Check sheet for the modelled part. Datum: model origin and axes. Units: mm. A direction names the side the tool comes from. Give positions to 0.01 mm unless a question says otherwise; leave off trailing zeros. Order: outer loops, then holes, each group sorted by start corner. A loop starts at its lowest first (then second) coordinate and runs counter-clockwise, first axis right, second up. Notation, with made-up numbers: (79.5, -28) -> (89.5, -28) arc R12 ccw to (89.5, -7) -> close; hole circle Ø5 at (13, 16). An arc over 180 degrees is marked (long way). One line per question, with ' | ' between items.
```python
from build123d import *

# Parameters (mm, degrees)
BOSS_EXTRUDE1_DEPTH = 350
BOSS_EXTRUDE2_DEPTH = 250
BOSS_EXTRUDE3_START = 250
BOSS_EXTRUDE3_DEPTH = 250
BOSS_EXTRUDE4_START = 350
SKETCH2_5_W         = 700
SKETCH2_5_H         = 50
BOSS_EXTRUDE4_DEPTH = 350
SKETCH3_R           = 100
CUT_EXTRUDE1_DEPTH  = 25


with BuildPart() as part:
    # Sketch2 → Boss-Extrude1 (new body)
    with BuildSketch(Plane.XY):
        with BuildLine():
            ThreePointArc((-86.602540378, -50), (-96.592582629, -25.88190451), (-100, 0))
            Line((-100, 0), (-720, 0))
            Line((-720, 0), (-720, -50))
            Line((-720, -50), (-86.602540378, -50))
        make_face()
        with BuildLine():
            Line((-20, 0), (-100, 0))
            ThreePointArc((-100, 0), (-96.592582629, -25.88190451), (-86.602540378, -50))
            Line((-86.602540378, -50), (-20, -50))
            Line((-20, -50), (-20, 0))
        make_face()
        with BuildLine():
            Line((0, 1020), (-50, 1020))
            Line((-50, 1020), (-100, 1020))
            ThreePointArc((-100, 1020), (-32.986729188, 522.100663541), (-50, 20))
            Line((-50, 20), (50, 20))
            ThreePointArc((50, 20), (67.013270812, 522.100663541), (0, 1020))
        make_face()
    extrude(amount=-BOSS_EXTRUDE1_DEPTH)

    # Sketch2_3 → Boss-Extrude2 (add)
    with BuildSketch(Plane.XY):
        with BuildLine():
            Line((0, 20), (0, -100))
            ThreePointArc((0, -100), (70.710678119, -70.710678119), (100, 0))
            ThreePointArc((100, 0), (88.519464769, 46.522084615), (56.713912861, 82.362200602))
            ThreePointArc((56.713912861, 82.362200602), (53.519940777, 51.163553411), (50, 20))
            Line((50, 20), (0, 20))
        make_face()
        with BuildLine():
            Line((0, 100), (0, 20))
            Line((0, 20), (50, 20))
            ThreePointArc((50, 20), (53.519940777, 51.163553411), (56.713912861, 82.362200602))
            ThreePointArc((56.713912861, 82.362200602), (29.696632299, 95.488795312), (0, 100))
        make_face()
        with BuildLine():
            ThreePointArc((-86.602540378, -50), (-50, -86.602540378), (0, -100))
            Line((0, -100), (0, 20))
            Line((0, 20), (-50, 20))
            ThreePointArc((-50, 20), (-46.044408297, 55.236219759), (-42.505548953, 90.516729438))
            ThreePointArc((-42.505548953, 90.516729438), (-84.411358523, 53.616439199), (-100, 0))
            Line((-100, 0), (-20, 0))
            Line((-20, 0), (-20, -50))
            Line((-20, -50), (-86.602540378, -50))
        make_face()
    extrude(amount=-BOSS_EXTRUDE2_DEPTH)

    # Sketch2_4 → Boss-Extrude3 (add)
    with BuildSketch(Plane.XY.offset(BOSS_EXTRUDE3_START)):
        with BuildLine():
            ThreePointArc((-86.602540378, -50), (67.847406367, -73.462435634), (56.713912861, 82.362200602))
            ThreePointArc((56.713912861, 82.362200602), (53.519940777, 51.163553411), (50, 20))
            Line((50, 20), (-50, 20))
            ThreePointArc((-50, 20), (-46.044408297, 55.236219759), (-42.505548953, 90.516729438))
            ThreePointArc((-42.505548953, 90.516729438), (-84.411358523, 53.616439199), (-100, 0))
            Line((-100, 0), (-20, 0))
            Line((-20, 0), (-20, -50))
            Line((-20, -50), (-86.602540378, -50))
        make_face()
    extrude(amount=-BOSS_EXTRUDE3_DEPTH)

    # Sketch2_5 → Boss-Extrude4 (add)
    with BuildSketch(Plane.XY.offset(BOSS_EXTRUDE4_START)):
        with BuildLine():
            Line((-50, 20), (50, 20))
            ThreePointArc((50, 20), (67.013270812, 522.100663541), (0, 1020))
            Line((0, 1020), (-100, 1020))
            ThreePointArc((-100, 1020), (-32.986729188, 522.100663541), (-50, 20))
        make_face()
        with Locations((-370, -25)):
            Rectangle(SKETCH2_5_W, SKETCH2_5_H)
    extrude(amount=-BOSS_EXTRUDE4_DEPTH)

    # Sketch3 → Cut-Extrude1 (cut)
    with BuildSketch(Plane.XZ.offset(50)):
        with Locations((-370, 0)):
            Circle(SKETCH3_R)
    extrude(amount=-CUT_EXTRUDE1_DEPTH, mode=Mode.SUBTRACT)


solid = part.part
```
Q1. Section check B-B (x = -370). Enter the section's corners in (y, z).
Result sheet:
outline: (-50, -350) -> (0, -350) -> (0, 350) -> (-50, 350) -> (-50, 100) -> (-25, 100) -> (-25, -100) -> (-50, -100) -> close
Q2. Section check D-D (x = -622). Enter the section's corners in (y, z).
Result sheet:
outline: (-50, -350) -> (0, -350) -> (0, 350) -> (-50, 350) -> close
Q3. Mould release check, pull along Y, two halves, no side actions. Record for faces 6 (the face through (3, 527, 350)), 7 (the face through (-371, -25, 1)), 8 (the face through (-83.984, 54.283, 3.5)), 9 (the face through (-33.347, 529.133, 4.9)): pulls with the +Y half, pulls with the -Y half, needs draft (parallel to the pull), parting line crosses it, or undercut.
Result sheet:
face 6: needs draft | face 7: pulls with the -Y half | face 8: undercut | face 9: undercut
Q4. Depth check by flat-ended pin: pin 1 Ø1.5 at (x, z) = (-380.5, 86) entering from +Y; pin 2 Ø5 at (x, z) = (-626.5, -269.5) entering from -Y; pin 3 Ø4 at (y, z) = (573.5, -174.5) entering from +X. Enter the tip coordinate at first touch or a pass-through.
Result sheet:
pin 1: stops at y = 0 | pin 2: stops at y = -50 | pin 3: stops at x = 64.13
Q5. Thickness scan on line 1 (Z direction, x = -370, y = -33); line 2 (Y direction, x = -380.5, z = -100); line 3 (X direction, y = 346, z = -110). Record the ranges inside material, lowest first.
Result sheet:
line 1: z = -350 to -100, 100 to 350 | line 2: y = -50 to 0 | line 3: x = -29.36 to 70.64
Q6. Section check A-A (z = 229.5). Enter the section's corners in (x, y).
Result sheet:
outline: (-720, -50) -> (-86.6, -50) arc R100 ccw (long way) to (56.71, 82.36) arc R3000 ccw to (0, 1020) -> (-100, 1020) arc R3000 cw to (-42.51, 90.52) arc R100 ccw to (-100, 0) -> (-720, 0) -> close
Q7. Access from +Z, -Z, +X, -X, +Y, -Y to the whole of each face (thin tool, end or side, straight path). Record for faces 1 (the face through (-20, -25, 301)), 2 (the face through (-449.357, -37.675, -60.848)), 3 (the face through (-20, -25, -299)), 4 (the face through (-1, 20, 301)), 5 (the face through (-1, 20, -299)).
Result sheet:
face 1: +Z, +X, -Y | face 2: -Y | face 3: -Z, +X, -Y | face 4: +Z, +X, -X | face 5: -Z, +X, -X
Q8. Section check C-C (y = 169). Enter the section's corners in (x, z), and give its area (3 significant figures).
Result sheet:
outline: (-36.14, -350) -> (63.86, -350) -> (63.86, 350) -> (-36.14, 350) -> close | area: 70,000 mm2
